```python
from build123d import *

# Parameters (mm, degrees)
F1_DEPTH = 25.4
F2_W     = 21.580409
F2_H     = 21.59
F3_DEPTH = 127
F5_DEPTH = 25.4


with BuildPart() as f1:
    # F0 (on Front) → F1 (new body)
    with BuildSketch(Plane.XZ):
        Polygon((-19.42512, -47.146455), (-44.815529, 63.343545), (-44.815529, -47.146455), align=None)
        Polygon((-19.42512, 63.343545), (-44.815529, 63.343545), (-19.42512, -47.146455), align=None)
    extrude(amount=F1_DEPTH)

    # F2 (on face) → F3 (cut)
    with BuildSketch(Plane.XY.offset(63.343545)):
        with Locations((-30.215324, -14.605)):
            Rectangle(F2_W, F2_H)
    extrude(amount=-F3_DEPTH, mode=Mode.SUBTRACT)

    # F4 (on face) → F5 (cut)
    with BuildSketch(Plane.XZ.offset(3.81)):
        Polygon((-19.42512, 63.343545), (-41.005529, 63.343545), (-19.42512, -47.146455), align=None)
    extrude(amount=-F5_DEPTH, mode=Mode.SUBTRACT)


solid = f1.part
```
Read the model definition and answer for the solid it produces. Units are mm, in the model's axes. A direction names the side the tool comes from. Round coordinates to 2 decimals unless told otherwise and drop trailing zeros. Write each loop counter-clockwise with the first axis right and the second up, starting at its lowest first coordinate (ties: lowest second). Pieces come first, ordered by that corner, then holes. Notation, with made-up numbers: (68, 57.5) - (80, 57.5) arc R33 cw to (80, 90.5) - close; hole circle Ø10 at (45, 66). An arc over 180 degrees is marked (long way). One line per item, written item: value.
Q1. Find section A-A (z = -27). Determine the outline of the cut face in (x, y), and give its area (3 significant figures).
The answers:
outline: (-44.82, -25.4) - (-41.01, -25.4) - (-41.01, -3.81) - (-23.36, -3.81) - (-23.36, 0) - (-44.82, 0) - close
area: 164 mm2
Q2. Each of these flat-tipped pins is pushed along its axis until it touches: P1, Ø4, axis at x = -32, z = -8, coming from the +Y side; P2, Ø4, axis at y = -12.5, z = -11.5, coming from the +X side; P3, Ø11, axis at x = -30.5, z = 2.5, coming from the -Y side; P4, Ø2, axis at x = -28.5, z = 7, coming from the -Y side. Where does it stop, or does it pass through?
The answers:
P1: stops at y = 0
P2: stops at x = -41.01
P3: stops at y = -3.81
P4: passes through
Q3. Find section B-B (y = -2). Determine the outline of the cut face in (x, z).
The answers:
outline: (-44.82, -47.15) - (-19.43, -47.15) - (-41.01, 63.34) - (-44.82, 63.34) - close
Q4. Find section D-D (z = 45). Determine the outline of the cut face in (x, y), and give its area (3 significant figures).
The answers:
outline: (-44.82, -25.4) - (-41.01, -25.4) - (-41.01, -3.81) - (-37.42, -3.81) - (-37.42, 0) - (-44.82, 0) - close
area: 110 mm2
Q5. Which of the six approach directions +Z, -Z, +X, -X, +Y, -Y give full straight-line access (tool end or side, diameter ignored) to faces 1 (the flat face through (-44.816, -13, 9)), 2 (the flat face through (-35, -3.81, -16))?
The answers:
face 1: +Z, -Z, -X, +Y, -Y
face 2: +Z, -Z, +X, -Y
Q6. Find section C-C (x = -35.75). Determine the outline of the cut face in (y, z).
The answers:
outline: (-3.81, -47.15) - (0, -47.15) - (0, 36.44) - (-3.81, 36.44) - close
Q7. Straight lines are drawn through the part: line 1 (X direction, y = -16.5, z = 12); line 2 (Y direction, x = -37, z = -16); line 3 (X direction, y = -3.5, z = 52.5). For each, find the intervals that lie inside material, in ascending order. Write a range as from..to.
The answers:
line 1: x = -44.82..-41.01
line 2: y = -3.81..0
line 3: x = -44.82..-38.89
